Geometry check sheet. Reference: the model listing, model coordinates, mm. Face numbers are marked on the shaded views. A direction names the side the tool comes from. Coordinates: 2 decimals unless noted, no trailing zeros. Order: outer loops, then holes, each group sorted by start corner. A loop starts at its lowest first (then second) coordinate and runs counter-clockwise, first axis right, second up. Notation, with made-up numbers: M -6.75,82.5 L 33.25,82.5 A24 cw 33.25,105.5 Z; hole C 54.25,-30 d8. An arc over 180 degrees is marked long. One line per item, written item: value. Start each with the question number.
1) Sectioned sample at D-D, the plane x = -4.5. Enter the section's corners in (y, z), then the cut area to 3 significant figures.
2) Sectioned sample at C-C, the plane z = -11. Enter the section's corners in (x, y), then the cut area to 3 significant figures.
3) Draft check along X on the marked faces 1, 2 and 3. Enter one of: pulls with the +X half, pulls with the -X half, needs draft (parallel to the pull), parting line crosses it, or undercut.
4) Sectioned sample at B-B, the plane x = 1.5. Enter the section's corners in (y, z), then the cut area to 3 significant figures.
5) Sectioned sample at A-A, the plane y = 7.5. Enter the section's corners in (x, z).
6) Access from +Z, -Z, +X, -X, +Y, -Y to the whole of each face (thin tool, end or side, straight path). Record for the marked faces 4 and 5.
7) Go/stop test with flat-tipped pins: P1, Ø1.8, axis at x = 0.46, y = 4, coming from the +Z side; P2, Ø1, axis at x = 0, y = 13, coming from the +Z side; P3, Ø1.5, axis at y = 2, z = -3, coming from the +X side. Record where each tip stops, or that it passes through.
8) Thickness scan on L1, parallel to X at y = 9.5, z = 1.25; L2, parallel to Z at x = 2, y = 7.5. Record the ranges inside material, lowest first. Write a range as from..to.
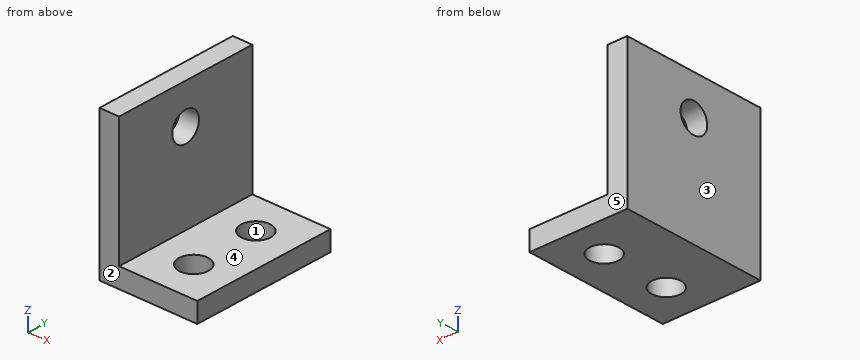
```python
from build123d import *

# Parameters (mm, degrees)
BOSS_EXTRUDE1_DEPTH             = 15
SKETCH3_R                       = 1.5
CUT_EXTRUDE1_DEPTH              = 3
SKETCH4_R                       = 1.5
SCHNITT_LINEAR_AUSTRAGEN1_DEPTH = 10


with BuildPart() as part:
    # Sketch1 → Boss-Extrude1 (new body)
    with BuildSketch(Plane(origin=(0, 0, 0), x_dir=(1, 0, 0), z_dir=(0, 1, 0))):
        Polygon((4.45631068, 12.597087379), (-5.54368932, 12.597087379), (-5.54368932, -2.402912621), (-3.54368932, -2.402912621), (-3.54368932, 10.597087379), (4.45631068, 10.597087379), align=None)
    extrude(amount=BOSS_EXTRUDE1_DEPTH)

    # Sketch3 → Cut-Extrude1 (cut, through all)
    with BuildSketch(Plane.XY.offset(-10.597087379)):
        with Locations((0.45631068, 11)):
            Circle(SKETCH3_R)
        with Locations((0.45631068, 4)):
            Circle(SKETCH3_R)
    extrude(amount=-CUT_EXTRUDE1_DEPTH, mode=Mode.SUBTRACT)

    # Sketch4 → Schnitt-Linear austragen1 (cut)
    with BuildSketch(Plane.ZY.offset(5.54368932)):
        with Locations((-1.597087379, 7.5)):
            Circle(SKETCH4_R)
    extrude(amount=-SCHNITT_LINEAR_AUSTRAGEN1_DEPTH, mode=Mode.SUBTRACT)


solid = part.part
```
Final values:
1. outline: M 0,-12.6 L 15,-12.6 L 15,2.4 L 0,2.4 Z; hole C 7.5,-1.6 d3
1. area: 218 mm^2
2. outline: M -5.54,0 L 4.46,0 L 4.46,15 L -5.54,15 Z; hole C 0.46,4 d3; hole C 0.46,11 d3
2. area: 136 mm^2
3. face 1: undercut
3. face 2: needs draft
3. face 3: pulls with the -X half
4. outline: M 0,-12.6 L 2.92,-12.6 L 2.92,-10.6 L 0,-10.6 Z; M 5.08,-12.6 L 9.92,-12.6 L 9.92,-10.6 L 5.08,-10.6 Z; M 12.08,-12.6 L 15,-12.6 L 15,-10.6 L 12.08,-10.6 Z
4. area: 21.4 mm^2
5. outline: M -5.54,-12.6 L 4.46,-12.6 L 4.46,-10.6 L -3.54,-10.6 L -3.54,-3.1 L -5.54,-3.1 Z; M -5.54,-0.1 L -3.54,-0.1 L -3.54,2.4 L -5.54,2.4 Z
6. face 4: +Z, +X, +Y, -Y
6. face 5: +Z, -Z, +X, -X, +Y
7. P1: passes through
7. P2: stops at z = -10.6
7. P3: stops at x = -3.54
8. L1: x = -5.54..-3.54
8. L2: z = -12.6..-10.6
